from build123d import *

# Parameters (mm, degrees)
F0_R     = 18.5
F0_R_2   = 11
F1_DEPTH = 7
F2_DEPTH = 1
F3_R     = 9
F4_DEPTH = 25


with BuildPart() as f1:
    # F0 (on Top) → F1 (new body)
    with BuildSketch(Plane.XY):
        Circle(F0_R)
        Circle(F0_R_2, mode=Mode.SUBTRACT)
    extrude(amount=F1_DEPTH)

    # F0 (on Top) → F2 (join)
    with BuildSketch(Plane.XY):
        Circle(F0_R)
        Circle(F0_R_2, mode=Mode.SUBTRACT)
        Circle(F0_R_2)
    extrude(amount=-F2_DEPTH)

    # F3 (on face) → F4 (cut)
    with BuildSketch(Plane(origin=(0, 0, -1), x_dir=(1, 0, 0), z_dir=(0, 0, -1))):
        Circle(F3_R)
    extrude(amount=-F4_DEPTH, mode=Mode.SUBTRACT)

    # F5 (on Front) → F6 (revolve, cut)
    with BuildSketch(Plane.XZ):
        Polygon((-18.5, 6.5), (-18.5, 0.5), (-15.5, 3.5), align=None)
    revolve(axis=Axis((0, 0, 3.0658829492), (0, 0, -1)), mode=Mode.SUBTRACT)


solid = f1.part
Read the model definition and answer for the solid it produces. Units are mm, in the model's axes. A direction names the side the tool comes from. Coordinates: 2 decimals unless noted, no trailing zeros. Write each loop counter-clockwise with the first axis right and the second up, starting at its lowest first coordinate (ties: lowest second). Pieces come first, ordered by that corner, then holes. Notation, with made-up numbers: M 29,-16 L 58,-16 A29 cw 58,12 Z; hole C 51,22 d4. An arc over 180 degrees is marked long. Use a Markdown table: item, result.
Q1. The part is cut by section C-C, the plane z = 5.5. Write down the section's boundary in (x, y), then the cut area to 3 significant figures.
Answer block:
| item | result |
|---|---|
| outline | C 0,0 d35; hole C 0,0 d22 |
| area | 582 mm2 |
Q2. Determine the mould class of faces 1 (the face through (-1.172, -8.923, -0.507)), 2 (the face through (-14.923, 4.7, 3.354)), 3 (the face through (3.9, 8.5, -1)) for opening direction Z: released by +Z, released by -Z, zero draft, split by the parting line, or undercut.
Answer block:
| item | result |
|---|---|
| face 1 | zero draft |
| face 2 | undercut |
| face 3 | released by -Z |
Q3. The part is cut by section A-A, the plane x = 0. Write down the section's boundary in (y, z), then the cut area to 3 significant figures.
Answer block:
| item | result |
|---|---|
| outline | M -18.5,-1 L -9,-1 L -9,0 L -11,0 L -11,7 L -18.5,7 L -18.5,6.5 L -15.5,3.5 L -18.5,0.5 Z; M 9,-1 L 18.5,-1 L 18.5,0.5 L 15.5,3.5 L 18.5,6.5 L 18.5,7 L 11,7 L 11,0 L 9,0 Z |
| area | 106 mm2 |
Q4. Each of these flat-tipped pins is pushed along its axis until it touches: pin 1 Ø14.5 at (x, y) = (0, 0) entering from +Z; pin 2 Ø2 at (x, z) = (-12.5, 3.5) entering from -Y. Where does it stop, or does it pass through?
Answer block:
| item | result |
|---|---|
| pin 1 | passes through |
| pin 2 | stops at y = -11.14 |
Q5. The part is cut by section D-D, the plane z = 3. Write down the section's boundary in (x, y), then the cut area to 3 significant figures.
Answer block:
| item | result |
|---|---|
| outline | C 0,0 d32; hole C 0,0 d22 |
| area | 424 mm2 |
Q6. Which of the six approach directions +Z, -Z, +X, -X, +Y, -Y give full straight-line access (tool end or side, diameter ignored) to faces 4 (the face through (3.401, -15.315, 3.688)), 5 (the face through (2, -9, 0)), 6 (the face through (8, -8, 7))?
Answer block:
| item | result |
|---|---|
| face 4 | none |
| face 5 | +Z |
| face 6 | +Z, +X, -X, +Y, -Y |
Q7. Straight lines are drawn through the part: L1, parallel to X at y = 0, z = -0.6; L2, parallel to Z at x = -2, y = -10; L3, parallel to Y at x = 9.5, z = 6.25. For each, find the intervals that lie inside material, in ascending order. Write a range as [from, to].
Answer block:
| item | result |
|---|---|
| L1 | x = [-18.5, -9], [9, 18.5] |
| L2 | z = [-1, 0] |
| L3 | y = [-15.58, -5.55], [5.55, 15.58] |
